```python
from build123d import *

# Parameters (mm, degrees)
BOSS_EXTRUDE1_DEPTH      = 65
SKETCH2_R                = 0.512371799
CUT_EXTRUDE1_DEPTH       = 3
M6_CLEARANCE_HOLE1_D     = 6.6
M6_CLEARANCE_HOLE1_DEPTH = 5
M6_CLEARANCE_HOLE1_TIP   = 1.982840043
M4_CLEARANCE_HOLE1_D     = 4.5
M4_CLEARANCE_HOLE1_DEPTH = 5
M4_CLEARANCE_HOLE1_TIP   = 1.351936393


with BuildPart() as part:
    # Sketch1 → Boss-Extrude1 (new body)
    with BuildSketch(Plane.XY):
        with BuildLine():
            Line((-16, -20), (16, -20))
            ThreePointArc((16, -20), (18.828427125, -18.828427125), (20, -16))
            Line((20, -16), (20, 16))
            ThreePointArc((20, 16), (18.828427125, 18.828427125), (16, 20))
            Line((16, 20), (-16, 20))
            ThreePointArc((-16, 20), (-18.828427125, 18.828427125), (-20, 16))
            Line((-20, 16), (-20, -16))
            ThreePointArc((-20, -16), (-18.828427125, -18.828427125), (-16, -20))
        make_face()
    extrude(amount=BOSS_EXTRUDE1_DEPTH)

    # Sketch2 → Cut-Extrude1 (cut)
    with BuildSketch(Plane(origin=(0, 0, 0), x_dir=(-1, 0, 0), z_dir=(0, 0, -1))):
        with Locations((-12.374368671, 12.374368671)):
            Circle(SKETCH2_R)
        with Locations((12.374368671, 12.374368671)):
            Circle(SKETCH2_R)
        with Locations((12.374368671, -12.374368671)):
            Circle(SKETCH2_R)
        with Locations((-12.374368671, -12.374368671)):
            Circle(SKETCH2_R)
    extrude(amount=-CUT_EXTRUDE1_DEPTH, mode=Mode.SUBTRACT)

    # M6 Clearance Hole1
    with Locations(Plane(origin=(0, 0, 0), x_dir=(-1, 0, 0), z_dir=(0, 0, -1))):
        with Locations((12.374368671, 12.374368671), (-12.374368671, 12.374368671), (-12.374368671, -12.374368671), (12.374368671, -12.374368671)):
            Hole(M6_CLEARANCE_HOLE1_D / 2, depth=M6_CLEARANCE_HOLE1_DEPTH)
            with Locations((0, 0, -(M6_CLEARANCE_HOLE1_DEPTH + M6_CLEARANCE_HOLE1_TIP / 2))):  # 118° drill point
                Cone(0, M6_CLEARANCE_HOLE1_D / 2, M6_CLEARANCE_HOLE1_TIP, mode=Mode.SUBTRACT)

    # M4 Clearance Hole1
    with Locations(Plane(origin=(20, 0, 0), x_dir=(0, 0, -1), z_dir=(1, 0, 0))):
        with Locations((-59.899999999, 0.460499028), (-39.899999999, 0.460499028)):
            Hole(M4_CLEARANCE_HOLE1_D / 2, depth=M4_CLEARANCE_HOLE1_DEPTH)
            with Locations((0, 0, -(M4_CLEARANCE_HOLE1_DEPTH + M4_CLEARANCE_HOLE1_TIP / 2))):  # 118° drill point
                Cone(0, M4_CLEARANCE_HOLE1_D / 2, M4_CLEARANCE_HOLE1_TIP, mode=Mode.SUBTRACT)


solid = part.part
```
The model under review builds one solid part; all positions refer to its coordinate system, in mm. A direction names the side the tool comes from. Give positions to 0.01 mm unless a question says otherwise; leave off trailing zeros. Answer in a Markdown table with one row per item.
Item 1: For line 1 along Y through (x, z) = (18.1, 59.9); line 2 along Y through (x, z) = (18, 48.5); line 3 along Z through (x, y) = (14.5, -13.5), list the stretches that pass through material, from the lowest coordinate up.
Check sheet entries:
| item | result |
|---|---|
| line 1 | -19.4 to -1.79, 2.71 to 19.4 |
| line 2 | -19.46 to 19.46 |
| line 3 | 5.54 to 65 |
Item 2: Tool access review of faces 1 (the face through (18.859, 18.797, 32.045)), 2 (the face through (17.46, -0.4, 41.98)), 3 (the face through (9.756, -14.382, 2.535)): name each direction out of +Z, -Z, +X, -X, +Y, -Y from which nothing blocks a thin tool from reaching the whole face with its end or side.
Check sheet entries:
| item | result |
|---|---|
| face 1 | +Z, -Z, +X, +Y |
| face 2 | +X |
| face 3 | -Z |
Item 3: Draft analysis for pull direction Y (two halves, no side actions). For faces 4 (the face through (-9.23, 13.37, 2.54)), 5 (the face through (0, 0, 0)), 6 (the face through (-18.797, 18.859, 32.045)), state which applies: +Y half, -Y half, draft (parallel to the pull), parting line (faces both ways), or undercut.
Check sheet entries:
| item | result |
|---|---|
| face 4 | undercut |
| face 5 | draft |
| face 6 | +Y half |
